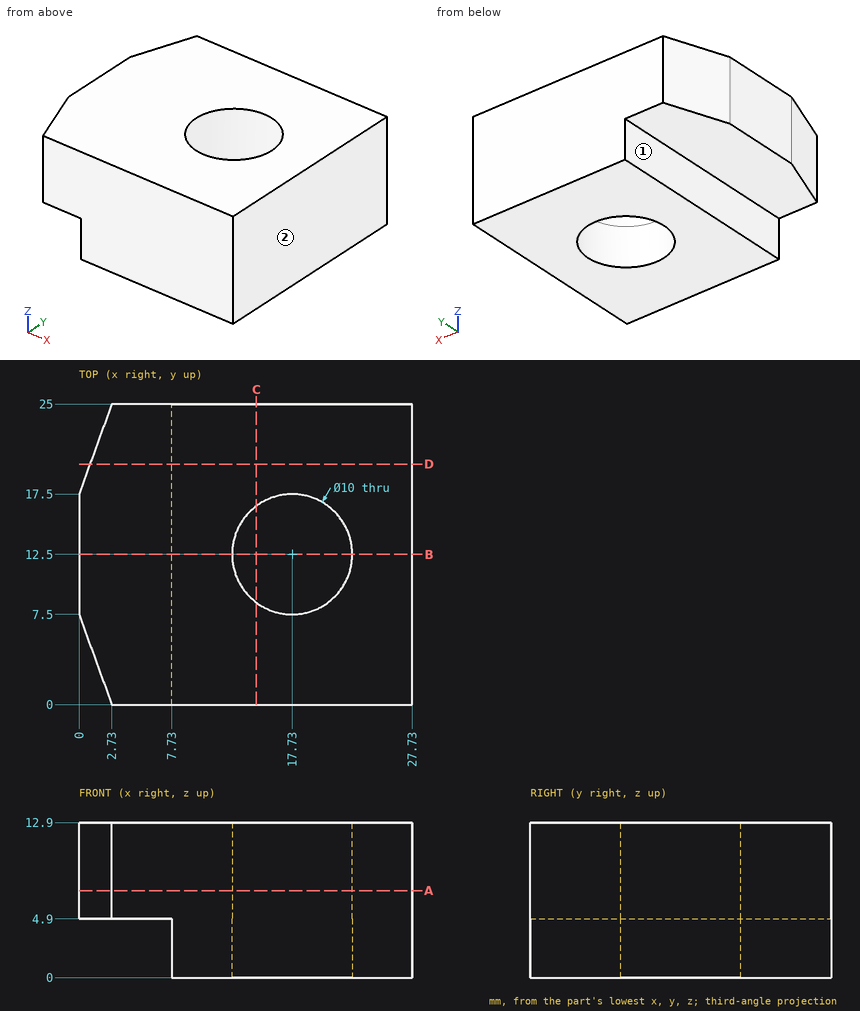
The drawing under review shows one solid part. Ordinate dimensions are in mm from its lowest x, y, z. A direction names the side the tool comes from. Coordinates: 2 decimals unless noted, no trailing zeros. Loops run counter-clockwise (first coordinate to the right, second up) from the corner with the lowest first, then second, coordinate; pieces in that order, holes last. Notation, with made-up numbers: (-25, -7) -> (21, -7) arc R31 ccw to (21, 17) -> close; hole circle Ø5 at (71.5, 49). An arc over 180 degrees is marked (long way). Answer as a JSON object with one key per item and string values.
Q1. Take a section at B-B on y = 12.5. Give the boundary of the cut face in (x, z), plus the area to 3 significant figures.
Answer block:
{"outline": "(0, 4.9) -> (7.73, 4.9) -> (7.73, 0) -> (12.73, 0) -> (12.73, 12.9) -> (0, 12.9) -> close; (22.73, 0) -> (27.73, 0) -> (27.73, 12.9) -> (22.73, 12.9) -> close", "area": "191 mm^2"}
Q2. Tool access review of the marked faces 1 and 2: name each direction out of +Z, -Z, +X, -X, +Y, -Y from which nothing blocks a thin tool from reaching the whole face with its end or side.
Answer block:
{"face 1": "-Z, -X, +Y, -Y", "face 2": "+Z, -Z, +X, +Y, -Y"}
Q3. Take a section at D-D on y = 20. Give the boundary of the cut face in (x, z), plus the area to 3 significant figures.
Answer block:
{"outline": "(0.91, 4.9) -> (7.73, 4.9) -> (7.73, 0) -> (27.73, 0) -> (27.73, 12.9) -> (0.91, 12.9) -> close", "area": "313 mm^2"}
Q4. Clearance check with flat-ended pins moving along their axes: pin 1 Ø2.5 at (y, z) = (7.5, 1.5) entering from -X; pin 2 Ø2.5 at (x, y) = (6, 12) entering from -Z. State where each tip first meets the part, or that it passes through.
Answer block:
{"pin 1": "stops at x = 7.73", "pin 2": "stops at z = 4.9"}
Q5. Take a section at C-C on x = 14.75. Give the boundary of the cut face in (y, z) (1 decimal).
Answer block:
{"outline": "(0, 0) -> (8.5, 0) -> (8.5, 12.9) -> (0, 12.9) -> close; (16.5, 0) -> (25, 0) -> (25, 12.9) -> (16.5, 12.9) -> close"}
Q6. Take a section at A-A on z = 7.25. Give the boundary of the cut face in (x, y).
Answer block:
{"outline": "(0, 7.5) -> (2.73, 0) -> (27.73, 0) -> (27.73, 25) -> (2.73, 25) -> (0, 17.5) -> close; hole circle Ø10 at (17.73, 12.5)"}
Q7. To check wall thickness, follow L1, parallel to Z at x = 2.75, y = 6.5; L2, parallel to X at y = 2, z = 0.5; L3, parallel to X at y = 14.5, z = 4.5. State the ranges of each line that lie inside material, in increasing order.
Answer block:
{"L1": "z = 4.9 to 12.9", "L2": "x = 7.73 to 27.73", "L3": "x = 7.73 to 13.15, 22.31 to 27.73"}
